Input: part model. Units: mm. Frame: model coordinates. A direction names the side the tool comes from. Round coordinates to 2 decimals unless told otherwise and drop trailing zeros. Loops run counter-clockwise (first coordinate to the right, second up) from the corner with the lowest first, then second, coordinate; pieces in that order, holes last.
1) First-contact query: pin 1 (1.5 mm diameter, centred on y = 35.5, z = 6.5, fed in from +X); pin 2 (3 mm diameter, centred on y = 55, z = 3, fed in from -X); pin 3 (3 mm diameter, centred on y = 32.5, z = 4.5, fed in from -X); pin 4 (16 mm diameter, centred on x = 0, y = 0, fed in from -Z). Flat tips, straight axial feed; report the tip coordinate or a pass-through.
2) Section A-A, the plane y = 0. Return loops of the section in (x, z), and give its area (3 significant figures).
3) Ray query, line 1 along Y through (x, z) = (0, 5.5); line 2 along X through (y, z) = (55, 9.5); line 3 along Y through (x, z) = (2.5, 5.25). Return the intervals inside material, ascending.
4) Draft query along Z for faces 1 (the face through (0, 58.848, 5)), 2 (the face through (0, 18, 10)), 3 (the face through (-0.89, -24.984, 4.93)). Return one class per face: pulls with the +Z half, pulls with the -Z half, needs draft (parallel to the pull), parting line crosses it, or undercut.
5) Access query for faces 4 (the face through (-0.1, 83.848, 1.6)), 5 (the face through (-7.5, 58, 5)), 6 (the face through (7.5, 58, 5)), 7 (the face through (-2.17, -9.76, 4.93)), 8 (the face through (0, 72, 8)). Directions: +Z, -Z, +X, -X, +Y, -Y. A direction counts if a zero-diameter tool reaches every point of the face in a straight line with its end or side. Return the directions, or none.
6) Section B-B, the plane x = 0. Return loops of the section in (y, z), and give its area (3 significant figures).
7) Section D-D, the plane y = 45. Return loops of the section in (x, z), and give its area (3 significant figures).
8) Section C-C, the plane x = -9. Return loops of the section in (y, z), and give its area (3 significant figures).
from build123d import *

# Parameters (mm, degrees)
SKETCH1_R           = 25
SKETCH1_R_2         = 10
BOSS_EXTRUDE1_DEPTH = 10
SKETCH2_W           = 15
SKETCH2_H           = 60
BOSS_EXTRUDE2_DEPTH = 10
FILLET1_R           = 15
SKETCH3_W           = 11
SKETCH3_H           = 6
CUT_EXTRUDE1_DEPTH  = 25


with BuildPart() as part:
    # Sketch1 → Boss-Extrude1 (new body)
    with BuildSketch(Plane.XY):
        Circle(SKETCH1_R)
        Circle(SKETCH1_R_2, mode=Mode.SUBTRACT)
    extrude(amount=BOSS_EXTRUDE1_DEPTH)

    # Sketch2 → Boss-Extrude2 (add)
    with BuildSketch(Plane.XY):
        with Locations((0, 53.848480035)):
            Rectangle(SKETCH2_W, SKETCH2_H)
    extrude(amount=BOSS_EXTRUDE2_DEPTH)

    # Fillet1
    fillet1_edges = [part.edges().sort_by_distance(p)[0] for p in [
        (-7.5, 23.848480035, 5),
        (7.5, 23.848480035, 5),
    ]]
    fillet(fillet1_edges, radius=FILLET1_R)

    # Sketch3 → Cut-Extrude1 (cut)
    with BuildSketch(Plane(origin=(0, 83.848480035, 0), x_dir=(1, 0, 0), z_dir=(0, 1, 0))):
        with Locations((0, -5)):
            Rectangle(SKETCH3_W, SKETCH3_H)
    extrude(amount=-CUT_EXTRUDE1_DEPTH, mode=Mode.SUBTRACT)


solid = part.part
Final values:
1. pin 1: stops at x = 7.5
1. pin 2: stops at x = -7.5
1. pin 3: stops at x = -7.64
1. pin 4: passes through
2. outline: (-25, 0) - (-10, 0) - (-10, 10) - (-25, 10) - close; (10, 0) - (25, 0) - (25, 10) - (10, 10) - close
2. area: 300 mm2
3. line 1: y = -25 to -10, 10 to 58.85
3. line 2: x = -7.5 to 7.5
3. line 3: y = -24.87 to -9.68, 9.68 to 58.85
4. face 1: undercut
4. face 2: pulls with the +Z half
4. face 3: needs draft
5. face 4: +Z, -Z, +X, -X, +Y
5. face 5: +Z, -Z, -X, +Y
5. face 6: +Z, -Z, +X, +Y
5. face 7: +Z, -Z
5. face 8: +Y
6. outline: (-25, 0) - (-10, 0) - (-10, 10) - (-25, 10) - close; (10, 0) - (83.85, 0) - (83.85, 2) - (58.85, 2) - (58.85, 8) - (83.85, 8) - (83.85, 10) - (10, 10) - close
6. area: 738 mm2
7. outline: (-7.5, 0) - (7.5, 0) - (7.5, 10) - (-7.5, 10) - close
7. area: 150 mm2
8. outline: (-23.32, 0) - (-4.36, 0) - (-4.36, 10) - (-23.32, 10) - close; (4.36, 0) - (26.53, 0) - (26.53, 10) - (4.36, 10) - close
8. area: 411 mm2
